```python
from build123d import *

# Parameters (mm, degrees)
SKETCH2_R           = 12
SKETCH2_R_2         = 7.5
SKETCH2_R_3         = 6.5
SKETCH2_R_4         = 4.75
BOSS_EXTRUDE2_DEPTH = 1
SKETCH2_4_R         = 7.5
SKETCH2_4_R_2       = 6.5
BOSS_EXTRUDE3_DEPTH = 3
BOSS_EXTRUDE4_START = 20
SKETCH2_5_R         = 12
SKETCH2_5_R_2       = 4.75
BOSS_EXTRUDE4_DEPTH = 20
CUT_EXTRUDE1_START  = -12.0000001
CUT_EXTRUDE1_DEPTH  = 24.0000001
CUT_EXTRUDE5_DEPTH  = 2
SKETCH11_W          = 15.5
SKETCH11_H          = 2
CUT_EXTRUDE6_DEPTH  = 18
THREAD2_PITCH       = 1


# Read off the part's stored shape, not the designer's step: Cut-Extrude1
with BuildPart() as part:
    # Sketch2 → Boss-Extrude2 (new body)
    # profile 1 of 3: a face of its own
    with BuildSketch(Plane(origin=(0, 0, 0), x_dir=(1, 0, 0), z_dir=(0, 1, 0))):
        with Locations(Location((0, 0, 0), (0, 0, 270))):
            Circle(SKETCH2_R)
        Circle(SKETCH2_R_2, mode=Mode.SUBTRACT)
    # profile 2 of 3: a face of its own
    with BuildSketch(Plane(origin=(0, 0, 0), x_dir=(1, 0, 0), z_dir=(0, 1, 0))):
        Circle(SKETCH2_R_2)
        Circle(SKETCH2_R_3, mode=Mode.SUBTRACT)
    # profile 3 of 3: a face of its own
    with BuildSketch(Plane(origin=(0, 0, 0), x_dir=(1, 0, 0), z_dir=(0, 1, 0))):
        Circle(SKETCH2_R_3)
        with Locations(Location((0, 0, 0), (0, 0, 270))):
            Circle(SKETCH2_R_4, mode=Mode.SUBTRACT)
    extrude(amount=-BOSS_EXTRUDE2_DEPTH)

    # Sketch2<4> → Boss-Extrude3 (add)
    with BuildSketch(Plane(origin=(0, 0, 0), x_dir=(1, 0, 0), z_dir=(0, 1, 0))):
        with Locations(Location((0, 0, 0), (0, 0, 270))):
            Circle(SKETCH2_4_R)
        with Locations(Location((0, 0, 0), (0, 0, 270))):
            Circle(SKETCH2_4_R_2, mode=Mode.SUBTRACT)
    extrude(amount=-BOSS_EXTRUDE3_DEPTH)

    # Sketch2<5> → Boss-Extrude4 (add)
    with BuildSketch(Plane(origin=(0, 0, 0), x_dir=(1, 0, 0), z_dir=(0, 1, 0)).offset(BOSS_EXTRUDE4_START)):
        with Locations(Location((0, 0, 0), (0, 0, 270))):
            Circle(SKETCH2_5_R)
        with Locations(Location((0, 0, 0), (0, 0, 270))):
            Circle(SKETCH2_5_R_2, mode=Mode.SUBTRACT)
    extrude(amount=-BOSS_EXTRUDE4_DEPTH)

    # Cut-Extrude1 outline → Cut-Extrude1 (cut)
    with BuildSketch(Plane(origin=(0, 0, 0), x_dir=(0, 0, -1), z_dir=(1, 0, 0)).offset(CUT_EXTRUDE1_START)):
        Polygon((-12, 20), (-12, 0), (12, 20), align=None)
    extrude(amount=CUT_EXTRUDE1_DEPTH, mode=Mode.SUBTRACT)

    # Sketch10 → Cut-Extrude5 (cut)
    with BuildSketch(Plane(origin=(0, 5.901639344, 4.918032787), x_dir=(1, 0, 0), z_dir=(0, 0.768221279597376, 0.6401843996644798))):
        with BuildLine():
            Line((-4.75, 6.401843997), (-7.75, 6.401843997))
            Line((-7.75, 6.401843997), (-7.75, -3.348156003))
            Line((-7.75, -3.348156003), (7.75, -3.348156003))
            Line((7.75, -3.348156003), (7.75, 6.401843997))
            Line((7.75, 6.401843997), (4.75, 6.401843997))
            add(Edge.make_bspline(
                [(-4.75, 6.401843997), (-4.75, 0.21872967), (0, 0.21872967), (4.75, 0.21872967), (4.75, 6.401843997)],
                knots=[1.570796327, 1.570796327, 1.570796327, 3.141592654, 3.141592654, 4.71238898, 4.71238898, 4.71238898], degree=2, weights=[1, 0.707106781, 1, 0.707106781, 1]))
        make_face()
        with BuildLine():
            Line((-7.75, 16.151843997), (-7.75, 6.401843997))
            Line((-7.75, 6.401843997), (-4.75, 6.401843997))
            add(Edge.make_bspline(
                [(0, 12.584958323), (-4.75, 12.584958323), (-4.75, 6.401843997)],
                knots=[0, 0, 0, 1.570796327, 1.570796327, 1.570796327], degree=2, weights=[1, 0.707106781, 1]))
            add(Edge.make_bspline(
                [(4.75, 6.401843997), (4.75, 12.584958323), (0, 12.584958323)],
                knots=[4.71238898, 4.71238898, 4.71238898, 6.283185307, 6.283185307, 6.283185307], degree=2, weights=[1, 0.707106781, 1]))
            Line((4.75, 6.401843997), (7.75, 6.401843997))
            Line((7.75, 6.401843997), (7.75, 16.151843997))
            Line((7.75, 16.151843997), (-7.75, 16.151843997))
        make_face()
    extrude(amount=-CUT_EXTRUDE5_DEPTH, mode=Mode.SUBTRACT)

    # Sketch11 → Cut-Extrude6 (cut)
    with BuildSketch(Plane(origin=(0, -2.143437241, 2.572124689), x_dir=(-1, 0, 0), z_dir=(0, 0.6401843996644799, -0.7682212795973757))):
        with Locations((0, 6.682212796)):
            Rectangle(SKETCH11_W, SKETCH11_H)
    extrude(amount=CUT_EXTRUDE6_DEPTH, mode=Mode.SUBTRACT)

    # Thread2: the profile of Thread Profile2 profile screwed along a right-hand helix of 2 turns, 8 arcs to a turn; built about Z, then put on its axis
    thread2_z = Axis((0, 0, 0), (0, 0, 1))
    thread2_corners = [(7.4997, 0, -0.000173205), (8.041265875, 0, 0.312499999), (8.041265875, 0, 0.437499999), (7.4997, 0, 0.750173202)]
    with BuildLine(mode=Mode.PRIVATE) as thread2_profile:
        Line(thread2_corners[0], thread2_corners[1])
        Line(thread2_corners[1], thread2_corners[2])
        Line(thread2_corners[2], thread2_corners[3])
        Line(thread2_corners[3], thread2_corners[0])
    thread2_cap = Face(thread2_profile.wire())
    thread2_turn_angles = [0, 22.5, 45, 67.5, 90, 112.5, 135, 157.5, 180, 202.5, 225, 247.5, 270, 292.5, 315, 337.5, 360]
    thread2_turn_weights = [1, 0.9238795325112867, 1, 0.9238795325112867, 1, 0.9238795325112867, 1, 0.9238795325112867, 1, 0.9238795325112867, 1, 0.9238795325112867, 1, 0.9238795325112867, 1, 0.9238795325112867, 1]
    thread2_turn_rails = [Edge.make_bspline([Vector(p[0], p[1], 0).rotate(thread2_z, thread2_turn_angles[k]) / thread2_turn_weights[k] + Vector(0, 0, p[2] + THREAD2_PITCH * thread2_turn_angles[k] / 360) for k in range(17)], [0, 0, 0, 1, 1, 2, 2, 3, 3, 4, 4, 5, 5, 6, 6, 7, 7, 8, 8, 8], 2, thread2_turn_weights) for p in thread2_corners]
    thread2_turn_sides = [Face.make_surface_from_curves(thread2_turn_rails[p[0]], thread2_turn_rails[p[1]]) for p in [(0, 1), (1, 2), (2, 3), (3, 0)]]
    thread2 = Plane(origin=(0, -3, 0), x_dir=(1, 0, 0), z_dir=(0, 1, 0)) * Solid(Shell([*[p.moved(Location((0, 0, THREAD2_PITCH * i))) for i in range(2) for p in thread2_turn_sides], thread2_cap, thread2_cap.rotate(thread2_z, 720).moved(Location((0, 0, THREAD2_PITCH * 720 / 360)))]))
    add(thread2)


solid = part.part
```
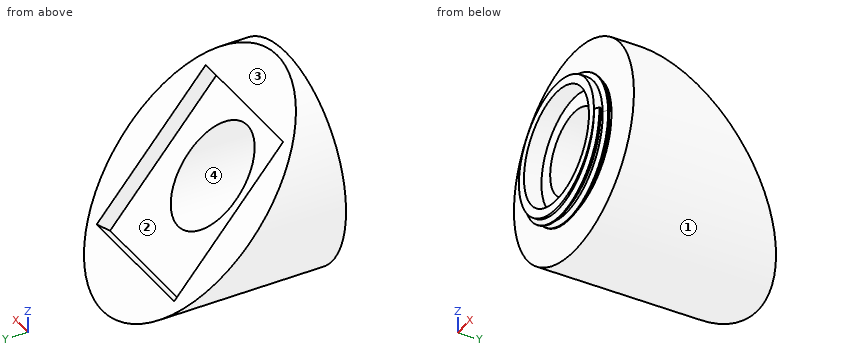
Here's how the part is built. I have some questions about the finished solid (model axes, mm). Face numbers are marked on the shaded views. Coordinates: 2 decimals unless noted, no trailing zeros. Loops run counter-clockwise (first coordinate to the right, second up) from the corner with the lowest first, then second, coordinate; pieces in that order, holes last. Notation, with made-up numbers: (19, 38) - (24, 38) arc R23 cw to (24, 52) - close; hole circle Ø9 at (-11.75, 72). An arc over 180 degrees is marked (long way). Return JSON: item names as keys, results as strings. Group by question number.
Item 1: I need wall thicknesses on line 1 (X direction, y = 2.5, z = 0); line 2 (X direction, y = 9, z = 0); line 3 (Y direction, x = -8.5, z = 7.5). Which ranges of each line are inside material? Lowest first, please. Write a range as from..to.
Item 2: If we section it at A-A on y = 5.25: Write out the boundary of the cut face in (x, z).
Item 3: If we section it at C-C on y = 1.75: Write out the boundary of the cut face in (x, z), and give its area (3 significant figures).
Item 4: Will these pins go through, and if not, where does the flat tip stop? P1, Ø5, axis at x = -4.5, z = -1.5, coming from the +Y side; P2, Ø4, axis at x = -2.5, z = -1, coming from the -Y side; P3, Ø1, axis at y = 6, z = -5, coming from the -X side; P4, Ø5, axis at x = 7.5, z = 5.5, coming from the +Y side.
Item 5: If we section it at D-D on z = 9.5: Write out the boundary of the cut face in (x, y), and give its area (3 significant figures).
Item 6: We'd pull the mould along Z, two halves only. Please class the marked faces 1, 2, 3 and 4: +Z half, -Z half, draft (parallel to the pull), parting line (faces both ways), or undercut.
Item 7: If we section it at B-B on x = -9.25: Write out the boundary of the cut face in (y, z), and give its area (3 significant figures).
Calculated:
{
 "1": {"line 1": "x = -12..-4.75, 4.75..12", "line 2": "x = -12..-7.75, 7.75..12", "line 3": "y = -1..3.75"},
 "2": {"outline": "(-10.56, 5.7) arc R12 ccw (long way) to (10.56, 5.7) - (7.75, 5.7) - (7.75, 2.58) - (3.99, 2.58) arc R4.75 cw (long way) to (-3.99, 2.58) - (-7.75, 2.58) - (-7.75, 5.7) - close"},
 "3": {"outline": "(-6.78, 9.9) arc R12 ccw (long way) to (6.78, 9.9) - close; hole circle Ø9.5 at (0, 0)", "area": "362 mm^2"},
 "4": {"P1": "stops at y = 10.73", "P2": "passes through", "P3": "stops at x = -11.12", "P4": "stops at y = 7.49"},
 "5": {"outline": "(-7.33, -1) - (7.33, -1) - (7.33, 2.08) - (-7.33, 2.08) - close", "area": "45.2 mm^2"},
 "6": {"face 1": "parting line", "face 2": "undercut", "face 3": "+Z half", "face 4": "undercut"},
 "7": {"outline": "(-1, -7.64) - (16.37, -7.64) - (3.63, 7.64) - (-1, 7.64) - close", "area": "168 mm^2"}
}
